The model under review builds one solid part; all positions refer to its coordinate system, in mm. Face numbers are marked on the shaded views. Round coordinates to 2 decimals unless told otherwise and drop trailing zeros. Write each loop counter-clockwise with the first axis right and the second up, starting at its lowest first coordinate (ties: lowest second). Pieces come first, ordered by that corner, then holes. Notation, with made-up numbers: (-8, 53.5) -> (10, 53.5) arc R33 cw to (10, 92.5) -> close; hole circle Ø7 at (3.25, 12.5). An arc over 180 degrees is marked (long way). Use CSV: the item, a comma, the result in double quotes. Start each with the question number.
1) Take a section at B-B, the plane x = 0. Give the boundary of the cut face in (y, z).
2) Mouldability with a two-part tool opening along Z and no side actions: class the marked faces 1, 2 and 3 as released by +Z, released by -Z, zero draft, split by the parting line, or undercut.
3) Wall thickness on probe 1 along Z at (x, y) = (0, -31.5); probe 2 along X at (y, z) = (-14, 1); probe 3 along Y at (x, z) = (1, -19): over which ranges is each line inside the solid? List them lowest first. Write a range as [from, to].
4) Take a section at A-A, the plane z = 0. Give the boundary of the cut face in (x, y).
5) For pin 1 Ø6 at (x, z) = (3.5, -3.5) entering from +Y; pin 2 Ø8 at (x, y) = (5.5, -78.5) entering from +Z; pin 3 Ø1.5 at (y, z) = (-63.5, 15.5) entering from +X; pin 4 Ø2 at (x, z) = (18.5, 1.5) entering from -Y, all flat-tipped, find the tip position at first contact; note any pin that passes through.
6) Take a section at C-C, the plane y = -51. Give the boundary of the cut face in (x, z).
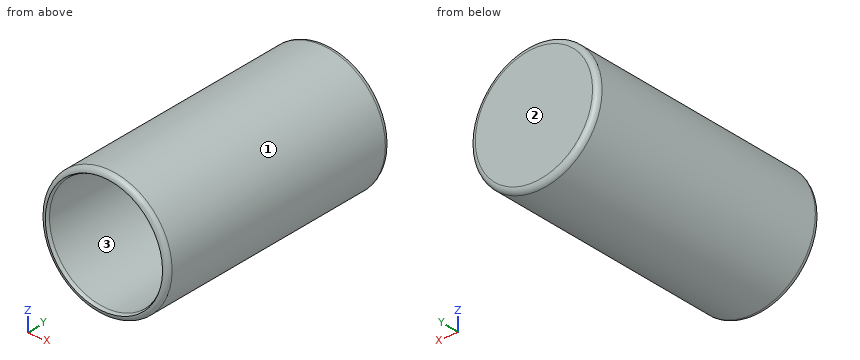
from build123d import *

# Parameters (mm, degrees)
F0_R     = 25
F1_DEPTH = 100
F2_T     = -2.5
F3_R     = 2


# Not quite as in the source:
# - a fillet or chamfer that OpenCascade refuses, or shapes differently, is made with other operations: its cross-section is extruded or revolved along the edge and cut away or added


with BuildPart() as f1:
    # F0 (on Front) → F1 (new body)
    with BuildSketch(Plane.XZ):
        Circle(F0_R)
    extrude(amount=F1_DEPTH)

    # F2
    f2_openings = [f1.faces().sort_by_distance(p)[0] for p in [
        (0, -100, 0),
    ]]
    offset(amount=F2_T, openings=f2_openings)

    # F3
    f3_edges = [f1.edges().sort_by_distance(p)[0] for p in [
        (25, -50, 0),
        (-25, 0, 0),
        (-25, -100, 0),
    ]]
    fillet(f3_edges, radius=F3_R)

    # F4: fillet of radius 2 on 3 edges, made by hand

    # F4_s1 → F4_t2 (revolve)
    with BuildSketch(Plane.XY):
        with BuildLine():
            ThreePointArc((22.5, -4.5), (21.9142135624, -3.0857864376), (20.5, -2.5))
            Line((20.5, -2.5), (22.5, -2.5))
            Line((22.5, -2.5), (22.5, -4.5))
        make_face()
    revolve(axis=Axis((0, -2.5, 0), (0, 1, 0)))

    # F4_s3 → F4_t4 (revolve, cut)
    with BuildSketch(Plane.XY):
        with BuildLine():
            ThreePointArc((23, -100), (22.6291713066, -99.3842311257), (22.5, -98.6771243445))
            Line((22.5, -98.6771243445), (22.5, -100))
            Line((22.5, -100), (23, -100))
        make_face()
    revolve(axis=Axis((0, -100, 0), (0, -1, 0)), mode=Mode.SUBTRACT)


solid = f1.part
Values found:
1,outline,"(-100, -23) arc R2 ccw to (-98, -25) -> (-2, -25) arc R2 ccw to (0, -23) -> (0, 23) arc R2 ccw to (-2, 25) -> (-98, 25) arc R2 ccw to (-100, 23) arc R2 ccw to (-98.68, 22.5) -> (-4.5, 22.5) arc R2 cw to (-2.5, 20.5) -> (-2.5, -20.5) arc R2 cw to (-4.5, -22.5) -> (-98.68, -22.5) arc R2 ccw to start"
2,face 1,"split by the parting line"
2,face 2,"zero draft"
2,face 3,"undercut"
3,probe 1,"[-25, -22.5], [22.5, 25]"
3,probe 2,"[-24.98, -22.48], [22.48, 24.98]"
3,probe 3,"[-2.5, 0]"
4,outline,"(-25, -98) arc R2 ccw to (-23, -100) arc R2 ccw to (-22.5, -98.68) -> (-22.5, -4.5) arc R2 cw to (-20.5, -2.5) -> (20.5, -2.5) arc R2 cw to (22.5, -4.5) -> (22.5, -98.68) arc R2 ccw to (23, -100) arc R2 ccw to (25, -98) -> (25, -2) arc R2 ccw to (23, 0) -> (-23, 0) arc R2 ccw to (-25, -2) -> close"
5,pin 1,"y = 0"
5,pin 2,"z = 24.95"
5,pin 3,"x = 20.19"
5,pin 4,"y = -2.5"
6,outline,"circle Ø50 at (0, 0); hole circle Ø45 at (0, 0)"
